Geometry: final body of the model. Coordinates: model frame, mm. A direction names the side the tool comes from. Give positions to 0.01 mm unless a question says otherwise; leave off trailing zeros. Order: outer loops, then holes, each group sorted by start corner. A loop starts at its lowest first (then second) coordinate and runs counter-clockwise, first axis right, second up. Notation, with made-up numbers: (50.25, 56.25) -> (98.25, 56.25) arc R23 cw to (98.25, 76.25) -> close; hole circle Ø2 at (64.25, 83.25). An arc over 180 degrees is marked (long way). One line per question, with ' | ' between items.
from build123d import *

# Parameters (mm, degrees)
SKETCH1_W           = 25
SKETCH1_H           = 25
SKETCH1_W_2         = 21
SKETCH1_H_2         = 21
BOSS_EXTRUDE1_DEPTH = 436.5
SKETCH2_R           = 1.5
CUT_EXTRUDE1_DEPTH  = 438.393987156
SKETCH3_R           = 1.5
CUT_EXTRUDE2_DEPTH  = 429


with BuildPart() as part:
    # Sketch1 → Boss-Extrude1 (new body)
    with BuildSketch(Plane.XY):
        Rectangle(SKETCH1_W, SKETCH1_H)
        Rectangle(SKETCH1_W_2, SKETCH1_H_2, mode=Mode.SUBTRACT)
    extrude(amount=-BOSS_EXTRUDE1_DEPTH)

    # Sketch2 → Cut-Extrude1 (cut, through all)
    with BuildSketch(Plane(origin=(0, 12.5, 0), x_dir=(1, 0, 0), z_dir=(0, 1, 0))):
        with Locations(Location((0, 366.5, 0), (0, 0, 270))):
            Circle(SKETCH2_R)
        with Locations(Location((0, 396.5, 0), (0, 0, 270))):
            Circle(SKETCH2_R)
        with Locations(Location((0, 426.5, 0), (0, 0, 270))):
            Circle(SKETCH2_R)
    cut_extrude1 = extrude(amount=-CUT_EXTRUDE1_DEPTH, mode=Mode.SUBTRACT)

    # Sketch3 → Cut-Extrude2 (cut)
    with BuildSketch(Plane(origin=(0, 12.5, 0), x_dir=(1, 0, 0), z_dir=(0, 1, 0))):
        Circle(SKETCH3_R)
    extrude(amount=-CUT_EXTRUDE2_DEPTH, mode=Mode.SUBTRACT)

    # Mirror1: Cut-Extrude1 across plane
    add(cut_extrude1.mirror(Plane.XY.offset(-218.25)), mode=Mode.SUBTRACT)


solid = part.part
1) Section A-A on y = 0.25. Return loops of the section in (x, z), plus the area to 3 significant figures.
Check result:
outline: (-12.5, -436.5) -> (-10.5, -436.5) -> (-10.5, 0) -> (-12.5, 0) -> close; (10.5, -436.5) -> (12.5, -436.5) -> (12.5, 0) -> (10.5, 0) -> close | area: 1,750 mm^2
2) Set-up query: faces 4 (the flat face through (10.5, 0, -215)), 5 (the flat face through (0, -12.5, -215)). Return all of +Z, -Z, +X, -X, +Y, -Y with unobstructed straight access to the full face (end or side cutting, diameter ignored); none if empty.
Check result:
face 4: +Z, -Z | face 5: +Z, -Z, +X, -X, -Y
3) Contact query for a flat-ended pin moving along its axis: pin 1 Ø2.5 at (x, z) = (0, -396.5) entering from +Y. Output: stop coordinate, or through.
Check result:
pin 1: passes through
4) Pull-direction query (X, two-part tool) for faces 1 (the flat face through (12.5, 0, -215)), 2 (the flat face through (-11, 0, -436.5)), 3 (the flat face through (0, 10.5, -215)); classes: +X half, -X half, draft (parallel to the pull), parting line (faces both ways), or undercut.
Check result:
face 1: +X half | face 2: draft | face 3: undercut
5) Section B-B on z = -384.5. Return loops of the section in (x, y).
Check result:
outline: (-12.5, -12.5) -> (12.5, -12.5) -> (12.5, 12.5) -> (-12.5, 12.5) -> close; hole (-10.5, -10.5) -> (10.5, -10.5) -> (10.5, 10.5) -> (-10.5, 10.5) -> close
6) Material intervals for probe 1 along X at (y, z) = (-6.5, -75.5); probe 2 along X at (y, z) = (11.35, -426.5), sorted ascending. Write a range as from..to.
Check result:
probe 1: x = -12.5..-10.5, 10.5..12.5 | probe 2: x = -12.5..-1.5, 1.5..12.5
